```python
from build123d import *

# Parameters (mm, degrees)
SKETCH1_R           = 18.5
SKETCH1_R_2         = 3.5
SKETCH1_R_3         = 2.25
BOSS_EXTRUDE1_DEPTH = 6
SKETCH2_R           = 3.75
CUT_EXTRUDE1_DEPTH  = 3.5
BOSS_EXTRUDE2_START = -6
BOSS_EXTRUDE2_DEPTH = 6
SKETCH4_W           = 62.93
SKETCH4_H           = 3
BOSS_EXTRUDE3_DEPTH = 85
SKETCH6_R           = 2
BOSS_EXTRUDE5_DEPTH = 6
SKETCH5_W           = 42
SKETCH5_H           = 44
SKETCH5_R           = 1.75
SKETCH5_R_2         = 3
BOSS_EXTRUDE4_DEPTH = 6
SKETCH7_W           = 15.07
SKETCH7_H           = 6
BOSS_EXTRUDE6_DEPTH = 3
CHAMFER1_SIZE       = 3
SKETCH8_W           = 6
SKETCH8_H           = 7
SKETCH8_W_2         = 18
SKETCH8_R           = 1.6
SKETCH8_W_3         = 19
BOSS_EXTRUDE7_DEPTH = 2.75
CHAMFER2_SIZE       = 7
FILLET1_R           = 5
CHAMFER3_SIZE       = 3


with BuildPart() as part:
    # Sketch1 → Boss-Extrude1 (new body)
    with BuildSketch(Plane.XY):
        Circle(SKETCH1_R)
        Circle(SKETCH1_R_2, mode=Mode.SUBTRACT)
        with Locations((-13.7, 0)):
            Circle(SKETCH1_R_3, mode=Mode.SUBTRACT)
        with Locations((13.7, 0)):
            Circle(SKETCH1_R_3, mode=Mode.SUBTRACT)
    extrude(amount=BOSS_EXTRUDE1_DEPTH)

    # Sketch2 → Cut-Extrude1 (cut)
    with BuildSketch(Plane.XY.offset(6)):
        with Locations((-13.7, 0)):
            Circle(SKETCH2_R)
        with Locations((13.7, 0)):
            Circle(SKETCH2_R)
    extrude(amount=-CUT_EXTRUDE1_DEPTH, mode=Mode.SUBTRACT)

    # Sketch3 → Boss-Extrude2 (add)
    with BuildSketch(Plane.XY.offset(6).offset(BOSS_EXTRUDE2_START)):
        with BuildLine():
            ThreePointArc((-15.5, -10.099504938), (-17.734147851, -5.267826876), (-18.5, 0))
            Line((-18.5, 0), (-18.5, -46.68))
            Line((-18.5, -46.68), (18.5, -46.68))
            Line((18.5, -46.68), (18.5, 0))
            ThreePointArc((18.5, 0), (17.734147851, -5.267826876), (15.5, -10.099504938))
            Line((15.5, -10.099504938), (15.5, -40.818554828))
            Line((15.5, -40.818554828), (15.5, -43.68))
            Line((15.5, -43.68), (13.738586173, -43.68))
            Line((13.738586173, -43.68), (-13.738586173, -43.68))
            Line((-13.738586173, -43.68), (-15.5, -43.68))
            Line((-15.5, -43.68), (-15.5, -40.818554828))
            Line((-15.5, -40.818554828), (-15.5, -10.099504938))
        make_face()
        with BuildLine():
            Line((-3, -20.512103215), (-15.5, -40.818554828))
            Line((-15.5, -40.818554828), (-15.5, -43.68))
            Line((-15.5, -43.68), (-13.738586173, -43.68))
            Line((-13.738586173, -43.68), (0, -21.361445172))
            Line((0, -21.361445172), (13.738586173, -43.68))
            Line((13.738586173, -43.68), (15.5, -43.68))
            Line((15.5, -43.68), (15.5, -40.818554828))
            Line((15.5, -40.818554828), (3, -20.512103215))
            Line((3, -20.512103215), (1.71251735, -18.420566884))
            ThreePointArc((1.71251735, -18.420566884), (0, -18.5), (-1.71251735, -18.420566884))
            Line((-1.71251735, -18.420566884), (-3, -20.512103215))
        make_face()
        with BuildLine():
            Line((3, -20.512103215), (3, -18.255136264))
            ThreePointArc((3, -18.255136264), (2.357710068, -18.349147207), (1.71251735, -18.420566884))
            Line((1.71251735, -18.420566884), (3, -20.512103215))
        make_face()
        with BuildLine():
            ThreePointArc((-1.71251735, -18.420566884), (-2.357710068, -18.349147207), (-3, -18.255136264))
            Line((-3, -18.255136264), (-3, -20.512103215))
            Line((-3, -20.512103215), (-1.71251735, -18.420566884))
        make_face()
    extrude(amount=BOSS_EXTRUDE2_DEPTH)

    # Sketch4 → Boss-Extrude3 (add)
    with BuildSketch(Plane.XY):
        with Locations((12.965, -45.18)):
            Rectangle(SKETCH4_W, SKETCH4_H)
    extrude(amount=BOSS_EXTRUDE3_DEPTH)

    # Sketch6 → Boss-Extrude5 (add)
    with BuildSketch(Plane(origin=(0, 0, 31), x_dir=(-1, 0, 0), z_dir=(0, 0, -1))):
        with BuildLine():
            Line((-44.43, -24.43), (-44.43, -43.68))
            Line((-44.43, -43.68), (33.57, -43.68))
            Line((33.57, -43.68), (33.57, -24.43))
            Line((33.57, -24.43), (-9.280986885, -24.43))
            ThreePointArc((-9.280986885, -24.43), (-20.68, -32.68), (-32.079013115, -24.43))
            Line((-32.079013115, -24.43), (-44.43, -24.43))
        make_face()
        with Locations((-32.43, -32.43)):
            Circle(SKETCH6_R, mode=Mode.SUBTRACT)
        with Locations((21.57, -32.43)):
            Circle(SKETCH6_R, mode=Mode.SUBTRACT)
    extrude(amount=BOSS_EXTRUDE5_DEPTH)

    # Sketch5 → Boss-Extrude4 (add)
    with BuildSketch(Plane.XY.offset(85)):
        with Locations((20.68, -21.68)):
            Rectangle(SKETCH5_W, SKETCH5_H)
        with Locations((5.18, -36.18)):
            Circle(SKETCH5_R, mode=Mode.SUBTRACT)
        with Locations((36.18, -36.18)):
            Circle(SKETCH5_R, mode=Mode.SUBTRACT)
        with Locations((5.18, -5.18)):
            Circle(SKETCH5_R, mode=Mode.SUBTRACT)
        with Locations((20.68, -20.68)):
            Circle(SKETCH5_R_2, mode=Mode.SUBTRACT)
        with Locations((36.18, -5.18)):
            Circle(SKETCH5_R, mode=Mode.SUBTRACT)
    extrude(amount=-BOSS_EXTRUDE4_DEPTH)

    # Sketch7 → Boss-Extrude6 (add)
    with BuildSketch(Plane.XZ.offset(46.68)):
        with Locations((-26.035, 28)):
            Rectangle(SKETCH7_W, SKETCH7_H)
    extrude(amount=-BOSS_EXTRUDE6_DEPTH)

    # Chamfer1
    chamfer1_edges = [part.edges().sort_by_distance(p)[0] for p in [
        (-18.5, -45.18, 31),
        (-18.5, -45.18, 25),
    ]]
    chamfer(chamfer1_edges, length=CHAMFER1_SIZE)

    # Sketch8 → Boss-Extrude7 (add)
    # profile 1 of 3: a face of its own
    with BuildSketch(Plane(origin=(44.43, 0, 0), x_dir=(0, 0, -1), z_dir=(1, 0, 0))):
        with Locations((-82, -40.18)):
            Rectangle(SKETCH8_W, SKETCH8_H)
    # profile 2 of 3: a face of its own
    with BuildSketch(Plane(origin=(44.43, 0, 0), x_dir=(0, 0, -1), z_dir=(1, 0, 0))):
        with Locations((-70, -40.18)):
            Rectangle(SKETCH8_W_2, SKETCH8_H)
        with Locations((-70, -40.68)):
            Circle(SKETCH8_R, mode=Mode.SUBTRACT)
    # profile 3 of 3: a face of its own
    with BuildSketch(Plane(origin=(44.43, 0, 0), x_dir=(0, 0, -1), z_dir=(1, 0, 0))):
        with Locations((-15.5, -40.18)):
            Rectangle(SKETCH8_W_3, SKETCH8_H)
        with Locations((-15.5, -40.68)):
            Circle(SKETCH8_R, mode=Mode.SUBTRACT)
    extrude(amount=-BOSS_EXTRUDE7_DEPTH)

    # Chamfer2
    # the kernel refuses this chamfer: 7 mm, written as the material it adds along each edge
    with BuildSketch(Plane(origin=(-0.32, -43.68, 85), x_dir=(-0.9996219169112968, -0.02749587661058612, 0), z_dir=(0, 0, -1)), Plane(origin=(18.5, -43.68, 0), x_dir=(0.9996219169112968, -0.027495876610586112, 0), z_dir=(0, 0, 1))) as chamfer2_piece_1:
        Polygon((CHAMFER2_SIZE * 0.999621916911, CHAMFER2_SIZE * 0.0274958766106), (-CHAMFER2_SIZE * 0.0274958766106, CHAMFER2_SIZE * 0.999621916911), (0, 0), align=None)
    extrude(amount=6)
    with BuildSketch(Plane(origin=(44.43, -43.68, 6), x_dir=(0, -0.02749587661058612, -0.9996219169112968), z_dir=(-1, 0, 0))) as chamfer2_piece_2_section:
        Polygon((CHAMFER2_SIZE * 0.999621916911, -CHAMFER2_SIZE * 0.0274958766106), (-CHAMFER2_SIZE * 0.0274958766106, -CHAMFER2_SIZE * 0.999621916911), (0, 0), align=None)
    chamfer2_piece_2 = extrude(amount=2.75, mode=Mode.PRIVATE)
    chamfer2_piece_2 = split(chamfer2_piece_2, bisect_by=Plane(origin=(43.055, -41.310788547, 0), z_dir=(0, 0, 1)), keep=Keep.TOP, mode=Mode.PRIVATE)
    chamfer2_piece_2 = split(chamfer2_piece_2, bisect_by=Plane(origin=(43.055, -36.68, 3.818532593), z_dir=(0, -1, 0)), keep=Keep.TOP, mode=Mode.PRIVATE)
    add(chamfer2_piece_2)
    with BuildSketch(Plane(origin=(44.43, -43.68, 61), x_dir=(0, -0.027495876610586126, -0.9996219169112968), z_dir=(-1, 0, 0))) as chamfer2_piece_3_section:
        Polygon((CHAMFER2_SIZE * 0.999621916911, -CHAMFER2_SIZE * 0.0274958766106), (-CHAMFER2_SIZE * 0.0274958766106, -CHAMFER2_SIZE * 0.999621916911), (0, 0), align=None)
    chamfer2_piece_3 = extrude(amount=2.75, mode=Mode.PRIVATE)
    chamfer2_piece_3 = split(chamfer2_piece_3, bisect_by=Plane(origin=(43.055, -36.68, 58.68717092), z_dir=(0, -1, 0)), keep=Keep.TOP, mode=Mode.PRIVATE)
    add(chamfer2_piece_3)

    # Fillet1
    fillet1_edges = [part.edges().sort_by_distance(p)[0] for p in [
        (44.43, -24.43, 28),
        (-33.57, -24.43, 28),
        (-0.32, 0.32, 82),
        (41.68, 0.32, 82),
        (-33.57, -46.68, 28),
    ]]
    fillet(fillet1_edges, radius=FILLET1_R)

    # Chamfer3
    # the kernel refuses this chamfer: 3 mm, written as the material it takes off along each edge
    with BuildSketch(Plane(origin=(-21.57, -32.43, 25), x_dir=(-1, 0, 0), z_dir=(0, -1, 0))) as chamfer3_piece_1:
        Polygon((2, -CHAMFER3_SIZE), (2 + CHAMFER3_SIZE, 0), (2, 0), align=None)
    revolve(axis=Axis((-21.57, -32.43, 25), (0, 0, -1)), mode=Mode.SUBTRACT)
    with BuildSketch(Plane(origin=(32.43, -32.43, 25), x_dir=(-1, 0, 0), z_dir=(0, -1, 0))) as chamfer3_piece_2:
        Polygon((2, -CHAMFER3_SIZE), (2 + CHAMFER3_SIZE, 0), (2, 0), align=None)
    revolve(axis=Axis((32.43, -32.43, 25), (0, 0, -1)), mode=Mode.SUBTRACT)


solid = part.part
```
Source: CAD feature listing. Evaluate the final solid. Frame: model axes, mm. A direction names the side the tool comes from. Give positions to 0.01 mm unless a question says otherwise; leave off trailing zeros. Write each loop counter-clockwise with the first axis right and the second up, starting at its lowest first coordinate (ties: lowest second). Pieces come first, ordered by that corner, then holes. Notation, with made-up numbers: (72.25, 15.25) - (81.25, 15.25) arc R18 cw to (81.25, 45.25) - close; hole circle Ø9 at (79.25, 54). An arc over 180 degrees is marked (long way). One line per item, written item: value. Start each with the question number.
Q1. Set-up query: faces 5 (the face through (-18.5, -45, 59)), 6 (the face through (3.233, -1.341, 2.958)), 7 (the face through (-10, -24.43, 28)). Return all of +Z, -Z, +X, -X, +Y, -Y with unobstructed straight access to the full face (end or side cutting, diameter ignored); none if empty.
Q2. Section query A-A, the plane z = 70. Return the cut outline in (x, y), then the cut area to 3 significant figures.
Q3. Draft query along X for faces 1 (the face through (-32.07, -25.86, 27.96)), 2 (the face through (-11.554, 0.676, 1.232)), 3 (the face through (17.164, -1.436, 4.274)), 4 (the face through (5, -36, 25)). Return one class per face: +X half, -X half, draft (parallel to the pull), parting line (faces both ways), or undercut.
Q4. Material intervals for probe 1 along Z at (x, y) = (34.5, -24.5); probe 2 along Y at (x, z) = (32.43, 29); probe 3 along Y at (x, z) = (9, 57), sorted ascending. Write a range as from..to.
Q5. Section query B-B, the plane z = 57.5. Return the cut outline in (x, y), then the cut area to 3 significant figures.
Q6. Section query C-C, the plane z = 48.5. Return the cut outline in (x, y).
Q7. First-contact query: pin 1 Ø1.9 at (y, z) = (-40.68, 70) entering from -X; pin 2 Ø6 at (x, y) = (-13.7, 0) entering from +Z; pin 3 Ø2 at (x, z) = (43.5, 16.5) entering from +Y; pin 4 Ø4 at (x, z) = (-16.5, 57) entering from +Y. Flat tips, straight axial feed; report the tip coordinate or a pass-through.
Answer:
1. face 5: +Z, -X, +Y, -Y
1. face 6: -Z
1. face 7: +X, -X, +Y
2. outline: (-18.5, -46.68) - (44.43, -46.68) - (44.43, -42.28) - (41.68, -42.28) - (41.68, -43.68) - (-18.5, -43.68) - close; (41.68, -39.08) - (44.43, -39.08) - (44.43, -36.68) - (41.68, -36.68) - close
2. area: 199 mm2
3. face 1: -X half
3. face 2: undercut
3. face 3: undercut
3. face 4: draft
4. probe 1: z = 25..31, 79..85
4. probe 2: y = -46.68..-34.43, -30.43..-24.43
4. probe 3: y = -46.68..-43.68
5. outline: (-18.5, -46.68) - (44.43, -46.68) - (44.43, -40.18) - (41.68, -40.18) - (41.68, -43.68) - (-18.5, -43.68) - close
5. area: 198 mm2
6. outline: (-18.5, -46.68) - (44.43, -46.68) - (44.43, -43.68) - (-18.5, -43.68) - close
7. pin 1: passes through
7. pin 2: stops at z = 2.5
7. pin 3: stops at y = -36.68
7. pin 4: stops at y = -43.68
